Can you work these out from the model? Positions are in its coordinate system, mm. Give positions to 0.01 mm unless a question says otherwise; leave off trailing zeros. Write each loop counter-clockwise with the first axis right and the second up, starting at its lowest first coordinate (ties: lowest second). Pieces come first, ordered by that corner, then holes.
```python
from build123d import *

# Parameters (mm, degrees)
BOSS_EXTRUDE1_DEPTH = 6.35
SKETCH2_R           = 11
SKETCH2_R_2         = 5.999988
CUT_EXTRUDE1_DEPTH  = 167.316670842


with BuildPart() as part:
    # Sketch1 → Boss-Extrude1 (new body)
    with BuildSketch(Plane(origin=(0, 0, 0), x_dir=(1, 0, 0), z_dir=(0, 1, 0))):
        Polygon((0, 0), (19.05, 0), (19.05, -6.35), (38.1, -6.35), (38.1, 0), (76.2, 0), (76.2, -6.35), (95.25, -6.35), (95.25, 0), (114.3, 0), (114.3, 114.3), (95.25, 114.3), (95.25, 120.65), (76.2, 120.65), (76.2, 114.3), (38.1, 114.3), (38.1, 120.65), (19.05, 120.65), (19.05, 114.3), (0, 114.3), (0, 95.25), (-6.35, 95.25), (-6.35, 76.2), (0, 76.2), (0, 38.1), (-6.35, 38.1), (-6.35, 19.05), (0, 19.05), align=None)
    extrude(amount=-BOSS_EXTRUDE1_DEPTH)

    # Sketch2 → Cut-Extrude1 (cut, through all)
    with BuildSketch(Plane(origin=(0, 0, 0), x_dir=(1, 0, 0), z_dir=(0, 1, 0))):
        with Locations(Location((88.3412, 57.15, 0), (0, 0, 270))):
            Circle(SKETCH2_R)
        with Locations(Location((41.275, 57.15, 0), (0, 0, 270))):
            Circle(SKETCH2_R_2)
    extrude(amount=-CUT_EXTRUDE1_DEPTH, mode=Mode.SUBTRACT)


solid = part.part
```
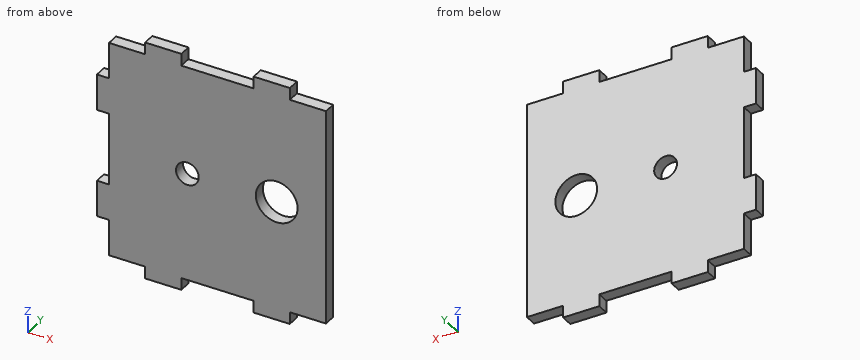
1) Suppose I cut it at D-D on z = -74. Write out the boundary of the cut face in (x, y), plus the area to 3 significant figures.
Values follow:
outline: (0, -6.35) - (114.3, -6.35) - (114.3, 0) - (0, 0) - close
area: 726 mm2
2) Suppose I cut it at C-C on x = 5.5. Write out the boundary of the cut face in (y, z).
Values follow:
outline: (-6.35, -114.3) - (0, -114.3) - (0, 0) - (-6.35, 0) - close
3) For pin 1 Ø9.5 at (x, z) = (41.275, -57.15) entering from +Y; pin 2 Ø3 at (x, y) = (12, -2.5) entering from -Z; pin 3 Ø1.9 at (y, z) = (-1.5, -13) entering from -X; pin 4 Ø3 at (y, z) = (-3, -119) entering from -X, each with a flat end and sliding along its axis, tell me the tip position at first contact or that it passes through.
Values follow:
pin 1: passes through
pin 2: stops at z = -114.3
pin 3: stops at x = 0
pin 4: stops at x = 19.05
4) Suppose I cut it at B-B on y = -1. State how many separate pieces and enclosed holes the cut face has, plus the area to 3 significant figures.
Values follow:
separate pieces: 1
enclosed holes: 2
area: 13,300 mm2
5) Please list where these lines run through material, in increasing order: L1, parallel to X at y = -1.25, z = -57.15; L2, parallel to X at y = -4.5, z = -75.5; L3, parallel to Z at x = 13, y = -5.5.
Values follow:
L1: x = 0 to 35.28, 47.27 to 77.34, 99.34 to 114.3
L2: x = 0 to 114.3
L3: z = -114.3 to 0
6) Suppose I cut it at A-A on z = -57.15. Write out the boundary of the cut face in (x, y).
Values follow:
outline: (0, -6.35) - (35.28, -6.35) - (35.28, 0) - (0, 0) - close; (47.27, -6.35) - (77.34, -6.35) - (77.34, 0) - (47.27, 0) - close; (99.34, -6.35) - (114.3, -6.35) - (114.3, 0) - (99.34, 0) - close
